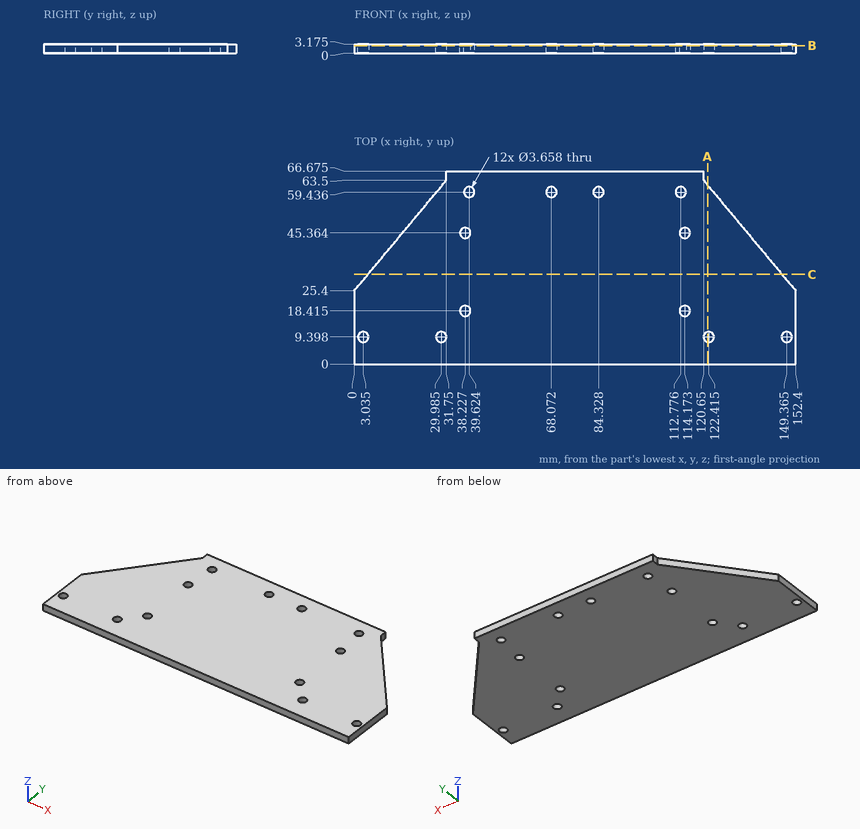
Geometry check sheet. Reference: drawing and pictorial views, mm from the part's lowest x, y, z. Give positions to 0.01 mm unless a question says otherwise; leave off trailing zeros. Write each loop counter-clockwise with the first axis right and the second up, starting at its lowest first coordinate (ties: lowest second). Pieces come first, ordered by that corner, then holes.
Item 1: Scan lines: L1, parallel to X at y = 44, z = 2 (1 decimal); L2, parallel to X at y = 46, z = 1.35 (1 decimal); L3, parallel to Y at x = 85.5, z = 0.95 (1 decimal). Record each from-to range of solid material in increasing order.
Item 2: Cross-section at B-B (z = 2.6). Count the separate pieces of the cut face and the enclosed holes in it, and give its area (3 significant figures).
Item 3: Cross-section at A-A (x = 122). Enter the section's corners in (y, z) (1 decimal).
Item 4: Gauge pin test, flat ends, axial feed: pin 1 (1.5 mm diameter, centred on y = 13.5, z = 2, fed in from -X); pin 2 (1 mm diameter, centred on y = 65, z = 1, fed in from +X). Record the tip position at first contact, or that the pin passes through.
Item 5: Cross-section at C-C (y = 31). Enter the section's corners in (x, z) (1 decimal).
Report:
1. L1: x = 15.5 to 37, 39.4 to 113, 115.4 to 136.9
1. L2: x = 17.2 to 36.5, 39.9 to 112.5, 115.9 to 135.2
1. L3: y = 0 to 58, 60.8 to 66.7
2. separate pieces: 1
2. enclosed holes: 12
2. area: 8,620 mm2
3. outline: (0, 0) - (7.6, 0) - (7.6, 3.2) - (0, 3.2) - close; (11.2, 0) - (61.9, 0) - (61.9, 3.2) - (11.2, 3.2) - close
4. pin 1: stops at x = 0
4. pin 2: stops at x = 120.65
5. outline: (4.7, 0) - (147.7, 0) - (147.7, 3.2) - (4.7, 3.2) - close
